Build history of the part. All positions in model axes, mm. A direction names the side the tool comes from. Round coordinates to 2 decimals unless told otherwise and drop trailing zeros. Loops run counter-clockwise (first coordinate to the right, second up) from the corner with the lowest first, then second, coordinate; pieces in that order, holes last.
from build123d import *

# Parameters (mm, degrees)
SKETCH1_W           = 80
SKETCH1_H           = 80
BOSS_EXTRUDE1_DEPTH = 45
SKETCH2_R           = 7.5
CUT_EXTRUDE1_DEPTH  = 122.757956619
SKETCH3_R           = 7.5
BOSS_EXTRUDE2_DEPTH = 300


with BuildPart() as part:
    # Sketch1 → Boss-Extrude1 (new body)
    with BuildSketch(Plane(origin=(0, 0, 0), x_dir=(1, 0, 0), z_dir=(0, 1, 0))):
        with Locations((-40, 40)):
            Rectangle(SKETCH1_W, SKETCH1_H)
    boss_extrude1 = extrude(amount=BOSS_EXTRUDE1_DEPTH)

    # Sketch2 → Cut-Extrude1 (cut, through all)
    with BuildSketch(Plane.XY):
        with Locations((-60, 22.5)):
            Circle(SKETCH2_R)
        with Locations((-20, 22.5)):
            Circle(SKETCH2_R)
    cut_extrude1 = extrude(amount=-CUT_EXTRUDE1_DEPTH, mode=Mode.SUBTRACT)

    # Sketch3 → Boss-Extrude2 (add)
    with BuildSketch(Plane(origin=(0, 0, 0), x_dir=(0, 0, -1), z_dir=(1, 0, 0))):
        with Locations(Location((20, 22.5, 0), (0, 0, 180))):
            Circle(SKETCH3_R)
        with Locations(Location((60, 22.5, 0), (0, 0, 180))):
            Circle(SKETCH3_R)
    extrude(amount=BOSS_EXTRUDE2_DEPTH)

    # Mirror3: Boss-Extrude1, Cut-Extrude1 across plane
    add(boss_extrude1.mirror(Plane(origin=(150, 0, 0), x_dir=(0, 0, 1), z_dir=(1, 0, 0))))
    add(cut_extrude1.mirror(Plane(origin=(150, 0, 0), x_dir=(0, 0, 1), z_dir=(1, 0, 0))), mode=Mode.SUBTRACT)


solid = part.part
(1) Slice it at A-A on y = 22.5. Count the separate pieces of the cut face and the enclosed holes in it, plus the area to 3 significant figures.
Responses:
separate pieces: 5
enclosed holes: 1
area: 17,000 mm2
(2) Which spindle directions (+Z, -Z, +X, -X, +Y, -Y) get a long thin tool onto all of the face, cutting with end or side? Do faces 5 (the face through (-41, 45, -41)), 6 (the face through (147.9, 17.4, -25.5)). Say none if no direction does.
Responses:
face 5: +Z, -Z, +X, -X, +Y
face 6: none
(3) Pull direction Y, two halves, no side cores. Call faces 1 (the face through (-60.976, 29.936, -39.44)), 2 (the face through (341, 0, -41)), 3 (the face through (341, 45, -41)), 4 (the face through (341, 22, -80)): +Y half, -Y half, draft (parallel to the pull), parting line (faces both ways), or undercut.
Responses:
face 1: undercut
face 2: -Y half
face 3: +Y half
face 4: draft
(4) Slice it at D-D on y = 4. List the corners of the cut face in (x, z).
Responses:
outline: (-80, -80) - (0, -80) - (0, 0) - (-80, 0) - close; (300, -80) - (380, -80) - (380, 0) - (300, 0) - close
(5) Pin check, flat tips, straight feed: P1, Ø17, axis at x = 360, y = 22.5, coming from the +Z side; P2, Ø10, axis at x = 182.5, z = -23, coming from the +Y side; P3, Ø3, axis at x = 180.5, y = 27, coming from the +Z side; P4, Ø6, axis at x = 122, z = -29, coming from the -Y side. Stop position of each tip, or through.
Responses:
P1: stops at z = 0
P2: stops at y = 30
P3: stops at z = -13.13
P4: stops at y = 18
(6) Slice it at C-C on x = -60. List the corners of the cut face in (y, z).
Responses:
outline: (0, -80) - (15, -80) - (15, 0) - (0, 0) - close; (30, -80) - (45, -80) - (45, 0) - (30, 0) - close
(7) Probe line 1 (X direction, y = 23.5, z = -36); line 2 (X direction, y = 8.5, z = -28); line 3 (Y direction, x = -20, z = -62). List the from-to ranges inside material, lowest first.
Responses:
line 1: x = -80 to -67.43, -52.57 to -27.43, -12.57 to 0, 300 to 312.57, 327.43 to 352.57, 367.43 to 380
line 2: x = -80 to 0, 300 to 380
line 3: y = 0 to 15, 30 to 45
(8) Slice it at B-B on z = -48. List the corners of the cut face in (x, y).
Responses:
outline: (-80, 0) - (0, 0) - (0, 45) - (-80, 45) - close; (300, 0) - (380, 0) - (380, 45) - (300, 45) - close; hole circle Ø15 at (-60, 22.5); hole circle Ø15 at (-20, 22.5); hole circle Ø15 at (320, 22.5); hole circle Ø15 at (360, 22.5)
